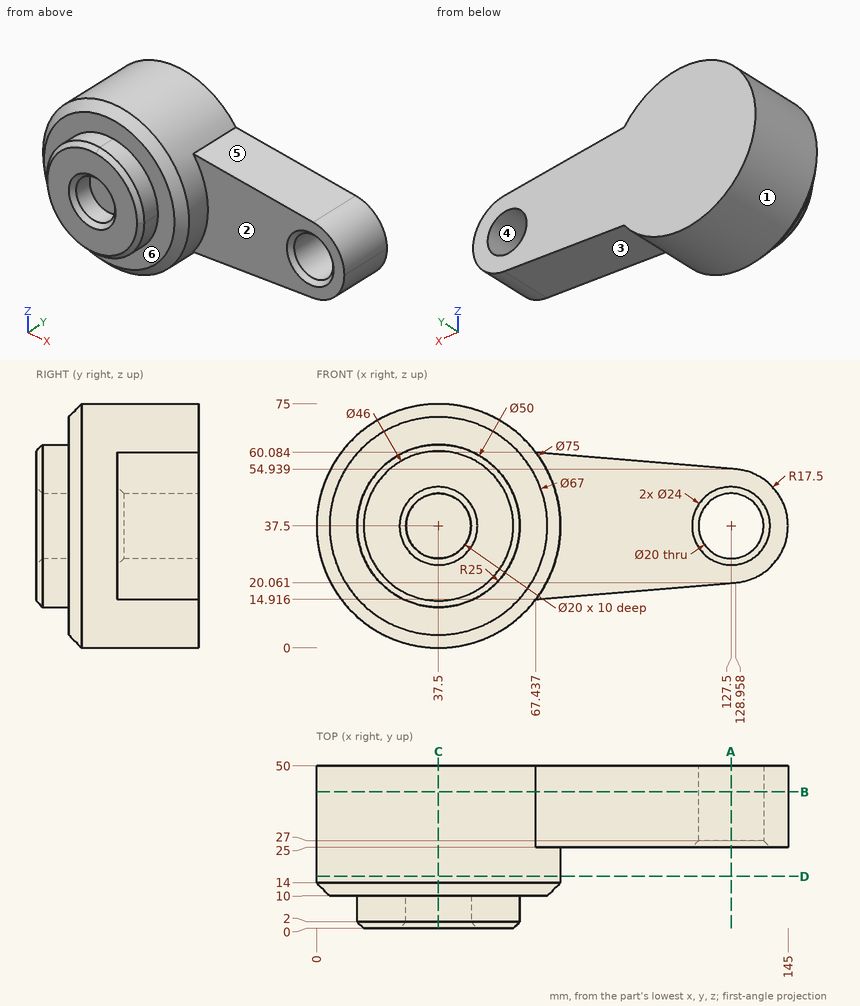
Answer from the drawing. Dimensions are ordinates in mm from the lowest x, y and z of the part. A direction names the side the tool comes from. Give positions to 0.01 mm unless a question says otherwise; leave off trailing zeros. Write each loop counter-clockwise with the first axis right and the second up, starting at its lowest first coordinate (ties: lowest second). Pieces come first, ordered by that corner, then holes. Notation, with made-up numbers: (76.5, 1) - (90.5, 1) arc R11 cw to (90.5, 13) - close; hole circle Ø6 at (52.25, 14.25). An arc over 180 degrees is marked (long way). Answer in a Markdown table with one row per item. Add a question column.
Item 1: Section D-D, the plane y = 16 is taken. Write down the section's boundary in (x, z), and give its area (3 significant figures).
Item 2: Section A-A, the plane x = 127.5 is taken. Write down the section's boundary in (y, z), and give its area (3 significant figures).
Item 3: Flat-ended cylindrical pins translate along their axes: P1, Ø5, axis at x = 53.5, y = 30, coming from the +Z side (1 decimal); P2, Ø1.5, axis at x = 54.5, z = 64.5, coming from the -Y side; P3, Ø23, axis at x = 37.5, z = 37.5, coming from the -Y side. Find the tip coordinate at first contact, or state that the pin passes through.
Item 4: Section B-B, the plane y = 42 is taken. Write down the section's boundary in (x, z), and give its area (3 significant figures).
Item 5: Find the intervals of material crossed by L1, parallel to X at y = 8.25, z = 37.5; L2, parallel to Z at x = 65.5, y = 33 (1 decimal), in increasing order.
Item 6: A tool of negligible diameter and unlimited length cuts with its end or side. For the marked faces 5 and 6, from which of +Z, -Z, +X, -X, +Y, -Y can it reach the whole face along a straight path? Write none if from no direction.
Item 7: Section C-C, the plane x = 37.5 is taken. Write down the section's boundary in (y, z).
Item 8: Determine the mould class of the marked faces 1, 2, 3 and 4 for opening direction Z: pulls with the +Z half, pulls with the -Z half, needs draft (parallel to the pull), parting line crosses it, or undercut.
Recorded:
| question | item | result |
|---|---|---|
| 1 | outline | circle Ø75 at (37.5, 37.5) |
| 1 | area | 4,420 mm2 |
| 2 | outline | (25, 19.94) - (50, 19.94) - (50, 27.5) - (27, 27.5) - (25, 25.5) - close; (25, 49.5) - (27, 47.5) - (50, 47.5) - (50, 55.06) - (25, 55.06) - close |
| 2 | area | 374 mm2 |
| 3 | P1 | stops at z = 72.5 |
| 3 | P2 | stops at y = 10 |
| 3 | P3 | stops at y = 0.5 |
| 4 | outline | (67.44, 14.92) - (128.96, 20.06) arc R17.5 ccw to (128.96, 54.94) - (67.44, 60.08) arc R37.5 ccw (long way) to start; hole circle Ø20 at (127.5, 37.5) |
| 4 | area | 6,760 mm2 |
| 5 | L1 | x = 12.5 to 27.5, 47.5 to 62.5 |
| 5 | L2 | z = 12.6 to 62.4 |
| 6 | face 5 | +Z, +X, +Y, -Y |
| 6 | face 6 | -Y |
| 7 | outline | (0, 14.5) - (2, 12.5) - (10, 12.5) - (10, 4) - (14, 0) - (50, 0) - (50, 75) - (14, 75) - (10, 71) - (10, 62.5) - (2, 62.5) - (0, 60.5) - (0, 49.5) - (2, 47.5) - (10, 47.5) - (10, 27.5) - (2, 27.5) - (0, 25.5) - close |
| 8 | face 1 | parting line crosses it |
| 8 | face 2 | needs draft |
| 8 | face 3 | pulls with the -Z half |
| 8 | face 4 | undercut |
